Read the model definition and answer for the solid it produces. Units are mm, in the model's axes. A direction names the side the tool comes from. Round coordinates to 2 decimals unless told otherwise and drop trailing zeros. Write each loop counter-clockwise with the first axis right and the second up, starting at its lowest first coordinate (ties: lowest second). Pieces come first, ordered by that corner, then holes. Notation, with made-up numbers: (-18, 44) -> (8, 44) arc R23 ccw to (8, 82) -> close; hole circle Ø6 at (0.5, 29). An arc over 180 degrees is marked (long way). Return JSON: item names as keys, results as strings.
from build123d import *

# Parameters (mm, degrees)
BOSS_EXTRUDE1_DEPTH      = 457.2
BOSS_EXTRUDE1_DEPTH_BACK = 457.2
SKETCH3_W                = 63.5
SKETCH3_H                = 31.75
SKETCH3_W_2              = 57.15
SKETCH3_H_2              = 25.4
SKETCH5_R                = 3.571875
CUT_EXTRUDE1_DEPTH       = 460.399570091
SKETCH6_R                = 6.35
CUT_EXTRUDE2_DEPTH       = 462.861565434


with BuildPart() as part:
    # Sketch3 → Boss-Extrude1 (new, two sides: drawn at the far end of the back side and taken through both)
    with BuildSketch(Plane.XY.offset(-BOSS_EXTRUDE1_DEPTH_BACK)):
        Rectangle(SKETCH3_W, SKETCH3_H)
        Rectangle(SKETCH3_W_2, SKETCH3_H_2, mode=Mode.SUBTRACT)
    extrude(amount=BOSS_EXTRUDE1_DEPTH + BOSS_EXTRUDE1_DEPTH_BACK)

    # Sketch5 → Cut-Extrude1 (cut, through all)
    with BuildSketch(Plane.XZ.offset(15.875)):
        with Locations(Location((-22.225, 392.1125, 0), (0, 0, 270))):
            Circle(SKETCH5_R)
        with Locations(Location((22.225, 392.1125, 0), (0, 0, 270))):
            Circle(SKETCH5_R)
        with Locations(Location((22.225, -392.1125, 0), (0, 0, 90))):
            Circle(SKETCH5_R)
        with Locations(Location((-22.225, -392.1125, 0), (0, 0, 90))):
            Circle(SKETCH5_R)
        with Locations(Location((22.225, 376.2375, 0), (0, 0, 90))):
            Circle(SKETCH5_R)
        with Locations(Location((-22.225, 376.2375, 0), (0, 0, 90))):
            Circle(SKETCH5_R)
        with Locations(Location((22.225, -376.2375, 0), (0, 0, 270))):
            Circle(SKETCH5_R)
        with Locations(Location((-22.225, -376.2375, 0), (0, 0, 270))):
            Circle(SKETCH5_R)
    extrude(amount=-CUT_EXTRUDE1_DEPTH, mode=Mode.SUBTRACT)

    # Sketch6 → Cut-Extrude2 (cut, through all)
    with BuildSketch(Plane.ZY.offset(31.75)):
        with Locations(Location((0, 0, 0), (0, 0, 270))):
            Circle(SKETCH6_R)
    extrude(amount=-CUT_EXTRUDE2_DEPTH, mode=Mode.SUBTRACT)


solid = part.part
Item 1: Section A-A (y = 0) is taken. Give the vertices of the cut face in (x, z) (3 decimals).
Worked answers:
{"outline": "(-31.75, -457.2) -> (-28.575, -457.2) -> (-28.575, -6.35) -> (-31.75, -6.35) -> close; (-31.75, 6.35) -> (-28.575, 6.35) -> (-28.575, 457.2) -> (-31.75, 457.2) -> close; (28.575, -457.2) -> (31.75, -457.2) -> (31.75, -6.35) -> (28.575, -6.35) -> close; (28.575, 6.35) -> (31.75, 6.35) -> (31.75, 457.2) -> (28.575, 457.2) -> close"}
Item 2: Section C-C (z = 364) is taken. Give the vertices of the cut face in (x, y) (3 decimals).
Worked answers:
{"outline": "(-31.75, -15.875) -> (31.75, -15.875) -> (31.75, 15.875) -> (-31.75, 15.875) -> close; hole (-28.575, -12.7) -> (28.575, -12.7) -> (28.575, 12.7) -> (-28.575, 12.7) -> close"}
Item 3: Straight lines are drawn through the part: L1, parallel to Y at x = -23, z = -21.5 (3 decimals); L2, parallel to X at y = -8, z = 400.5 (3 decimals); L3, parallel to Z at x = 21, y = 14. For each, find the intervals that lie inside material, in ascending order. Write a range as [from, to].
Worked answers:
{"L1": "y = [-15.875, -12.7], [12.7, 15.875]", "L2": "x = [-31.75, -28.575], [28.575, 31.75]", "L3": "z = [-457.2, -395.47], [-388.76, -379.59], [-372.88, 372.88], [379.59, 388.76], [395.47, 457.2]"}
Item 4: Section B-B (x = 11) is taken. Give the vertices of the cut face in (y, z) (3 decimals).
Worked answers:
{"outline": "(-15.875, -457.2) -> (-12.7, -457.2) -> (-12.7, 457.2) -> (-15.875, 457.2) -> close; (12.7, -457.2) -> (15.875, -457.2) -> (15.875, 457.2) -> (12.7, 457.2) -> close"}
Item 5: For a pull along X with two mould halves and no side action, classify faces 3 (the flat face through (0, -15.875, -6)), 4 (the flat face through (-31.75, 3, -6)), 5 (the flat face through (0, -12.7, -6)) as released by +X, released by -X, zero draft, split by the parting line, or undercut.
Worked answers:
{"face 3": "zero draft", "face 4": "released by -X", "face 5": "undercut"}
Item 6: A tool of negligible diameter and unlimited length cuts with its end or side. For faces 1 (the flat face through (0, 12.7, -6)), 2 (the flat face through (0, 15.875, -6)), from which of +Z, -Z, +X, -X, +Y, -Y can it reach the whole face along a straight path? Write none if from no direction.
Worked answers:
{"face 1": "+Z, -Z", "face 2": "+Z, -Z, +X, -X, +Y"}
Item 7: A flat-ended cylindrical pin translates along its axis: pin 1 (9.5 mm diameter, centred on x = -22.22, z = 392.11, fed in from +Y) (3 decimals). Find the tip coordinate at first contact, or state that the pin passes through.
Worked answers:
{"pin 1": "stops at y = 15.875"}
